Geometry check sheet. Reference: the model listing, model coordinates, mm. A direction names the side the tool comes from. Give positions to 0.01 mm unless a question says otherwise; leave off trailing zeros. Write each loop counter-clockwise with the first axis right and the second up, starting at its lowest first coordinate (ties: lowest second). Pieces come first, ordered by that corner, then holes. Notation, with made-up numbers: (8.25, 39.25) - (40.25, 39.25) arc R21 cw to (40.25, 62.25) - close; hole circle Ø10 at (-18, 39). An arc over 180 degrees is marked (long way). Write item = value, one per line. Start each with the question number.
(1) Draft check along Z on faces 1 (the cylindrical face through (23.19, -11.51, 7.57)), 2 (the flat face through (-18, 4, 41.144)), 3 (the cylindrical face through (-18.07, -11.4, 20.86)). Enter one of: pulls with the +Z half, pulls with the -Z half, needs draft (parallel to the pull), parting line crosses it, or undercut.
(2) Depth check by flat-ended pin: pin 1 Ø1.5 at (y, z) = (52.5, 6.5) entering from -X; pin 2 Ø1.1 at (x, z) = (-3.5, 0.5) entering from +Y; pin 3 Ø6 at (x, z) = (25, 34.14) entering from -Y; pin 4 Ø1 at (x, y) = (-15.5, 38.5) entering from -Z. Enter the tip coordinate at first touch or a pass-through.
(3) Thickness scan on L1, parallel to X at y = 0.5, z = 37; L2, parallel to Y at x = -28, z = 20.5; L3, parallel to Z at x = -8.5, y = 0.5. Record the ranges inside material, lowest first.
(4) Section check A-A, the plane y = 12. Enter the section's corners in (x, z).
(5) Section check D-D, the plane z = 14.5. Enter the section's corners in (x, y), plus the area to 3 significant figures.
(6) Section check B-B, the plane x = 25. Enter the section's corners in (y, z).
(7) Section check C-C, the plane y = 3. Enter the section's corners in (x, z).
(8) Access from +Z, -Z, +X, -X, +Y, -Y to the whole of each face (thin tool, end or side, straight path). Record for faces 4 (the cylindrical face through (18.1, -11.43, 20.86)), 5 (the flat face through (17.5, 25, 21)), 6 (the flat face through (33, -11, 21)), 7 (the cylindrical face through (-17.99, 26.79, 21.36)), 8 (the flat face through (-18.5, 25, 17)).
```python
from build123d import *

# Parameters (mm, degrees)
BASE_FLANGE1_DEPTH         = 1
SKETCHED_START             = -40
SKETCHED_BEND3_OUTLINE_W   = 40
SKETCHED_BEND3_OUTLINE_H   = 1
SKETCHED_BEND3_DEPTH       = 28.18876
SKETCHED_START_2           = -11.4496
SKETCHED_BEND3_2_DEPTH     = 0.4496
SKETCHED_START_3           = -12
SKETCHED_BEND3_3_DEPTH     = 2
SKETCHED_START_4           = -60
SKETCHED_BEND3_4_DEPTH     = 120
SKETCHED_BEND7_DEPTH       = 72
SKETCHED_START_5           = -10
SKETCHED_BEND7_2_OUTLINE_W = 1
SKETCHED_BEND7_2_OUTLINE_H = 40
SKETCHED_BEND7_2_DEPTH     = 55
SKETCHED_BEND7_3_DEPTH     = 20
SKETCHED_BEND7_4_DEPTH     = 2
SKETCHED_START_6           = 45
SKETCHED_BEND7_5_OUTLINE_W = 1
SKETCHED_BEND7_5_OUTLINE_H = 40
SKETCHED_BEND7_5_DEPTH     = 15
SKETCHED_START_7           = 1.14380551
SKETCHED_BEND7_6_DEPTH     = 40
SKETCHED_START_8           = -42.14380551
SKETCHED_BEND7_7_DEPTH     = 84.28761102
SKETCH9_R                  = 3
CUT_EXTRUDE1_DEPTH         = 98.989397047
F_4_CLEARANCE_HOLE1_D      = 3.2639
F_4_CLEARANCE_HOLE1_DEPTH  = 10
F_4_CLEARANCE_HOLE1_TIP    = 0.980574487
F_6_CLEARANCE_HOLE1_D      = 3.7973
F_6_CLEARANCE_HOLE2_D      = 3.7973


with BuildPart() as part:
    # Base-Flange1: sheet metal written as solids
    # Sketch1 → Base-Flange1 (new body)
    with BuildSketch(Plane.XY):
        with BuildLine():
            Line((-19, -10), (-19, -35))
            ThreePointArc((-19, -35), (-20.464466094, -38.535533906), (-24, -40))
            Line((-24, -40), (-54, -40))
            ThreePointArc((-54, -40), (-57.535533906, -38.535533906), (-59, -35))
            Line((-59, -35), (-59, 45))
            ThreePointArc((-59, 45), (-54.606601718, 55.606601718), (-44, 60))
            Line((-44, 60), (-34, 60))
            ThreePointArc((-34, 60), (-23.393398282, 55.606601718), (-19, 45))
            Line((-19, 45), (-19, 10))
            Line((-19, 10), (19, 10))
            Line((19, 10), (19, 45))
            ThreePointArc((19, 45), (23.393398282, 55.606601718), (34, 60))
            Line((34, 60), (44, 60))
            ThreePointArc((44, 60), (54.606601718, 55.606601718), (59, 45))
            Line((59, 45), (59, -35))
            ThreePointArc((59, -35), (57.535533906, -38.535533906), (54, -40))
            Line((54, -40), (24, -40))
            ThreePointArc((24, -40), (20.464466094, -38.535533906), (19, -35))
            Line((19, -35), (19, -10))
            Line((19, -10), (-19, -10))
        make_face()
    extrude(amount=-BASE_FLANGE1_DEPTH)

    # Sketched Bend3: read off the stored shape, not the designer's step
    # Sketched Bend3 outline → Sketched Bend3 (cut)
    with BuildSketch(Plane(origin=(0, 0, 0), x_dir=(1, 0, 0), z_dir=(0, 1, 0)).offset(SKETCHED_START)):
        with Locations((-39, 0.5)):
            Rectangle(SKETCHED_BEND3_OUTLINE_W, SKETCHED_BEND3_OUTLINE_H)
        with Locations((39, 0.5)):
            Rectangle(SKETCHED_BEND3_OUTLINE_W, SKETCHED_BEND3_OUTLINE_H)
    extrude(amount=SKETCHED_BEND3_DEPTH, mode=Mode.SUBTRACT)

    # Sketched Bend3 2 outline → Sketched Bend3 2 (add)
    with BuildSketch(Plane(origin=(0, 0, 0), x_dir=(1, 0, 0), z_dir=(0, 1, 0)).offset(SKETCHED_START_2)):
        with BuildLine():
            Line((-19, 1), (-19, 24.64380551))
            ThreePointArc((-19, 24.64380551), (-20.464466094, 28.179339416), (-24, 29.64380551))
            Line((-24, 29.64380551), (-54, 29.64380551))
            ThreePointArc((-54, 29.64380551), (-57.535533906, 28.179339416), (-59, 24.64380551))
            Line((-59, 24.64380551), (-59, 1))
            Line((-59, 1), (-19, 1))
        make_face()
        with BuildLine():
            Line((19, 24.64380551), (19, 1))
            Line((19, 1), (59, 1))
            Line((59, 1), (59, 24.64380551))
            ThreePointArc((59, 24.64380551), (57.535533906, 28.179339416), (54, 29.64380551))
            Line((54, 29.64380551), (24, 29.64380551))
            ThreePointArc((24, 29.64380551), (20.464466094, 28.179339416), (19, 24.64380551))
        make_face()
    extrude(amount=SKETCHED_BEND3_2_DEPTH)

    # Sketched Bend3 3 outline → Sketched Bend3 3 (add)
    with BuildSketch(Plane(origin=(0, 0, 0), x_dir=(1, 0, 0), z_dir=(0, 1, 0)).offset(SKETCHED_START_3)):
        with BuildLine():
            Line((-19, 1), (-19, 24.64380551))
            ThreePointArc((-19, 24.64380551), (-20.464466094, 28.179339416), (-24, 29.64380551))
            Line((-24, 29.64380551), (-54, 29.64380551))
            ThreePointArc((-54, 29.64380551), (-57.535533906, 28.179339416), (-59, 24.64380551))
            Line((-59, 24.64380551), (-59, 1))
            Line((-59, 1), (-19, 1))
        make_face()
        with BuildLine():
            ThreePointArc((59, 24.64380551), (57.535533906, 28.179339416), (54, 29.64380551))
            Line((54, 29.64380551), (24, 29.64380551))
            ThreePointArc((24, 29.64380551), (20.464466094, 28.179339416), (19, 24.64380551))
            Line((19, 24.64380551), (19, 1))
            Line((19, 1), (59, 1))
            Line((59, 1), (59, 24.64380551))
        make_face()
    extrude(amount=SKETCHED_BEND3_3_DEPTH)

    # Sketched Bend3 4 outline → Sketched Bend3 4 (cut)
    with BuildSketch(Plane.YZ.offset(SKETCHED_START_4)):
        with BuildLine():
            Line((-11, -2), (-11, -29.64380551))
            Line((-11, -29.64380551), (-10, -29.64380551))
            Line((-10, -29.64380551), (-10, -1))
            ThreePointArc((-10, -1), (-10.707106781, -1.292893219), (-11, -2))
        make_face()
        with BuildLine():
            Line((-12, -1), (-12, -2))
            ThreePointArc((-12, -2), (-11.414213562, -0.585786438), (-10, 0))
            Line((-10, 0), (-11.81124, 0))
            Line((-11.81124, 0), (-11.81124, -1))
            Line((-11.81124, -1), (-12, -1))
        make_face()
    extrude(amount=SKETCHED_BEND3_4_DEPTH, mode=Mode.SUBTRACT)

    # Sketched Bend7: read off the stored shape, not the designer's step
    # Sketched Bend7 outline → Sketched Bend7 (cut)
    with BuildSketch(Plane(origin=(0, 0, 0), x_dir=(1, 0, 0), z_dir=(0, 1, 0)).offset(SKETCHED_START_3)):
        with BuildLine():
            ThreePointArc((-18.232050807, 0), (-17.5, 0.732050807), (-16.5, 1))
            Line((-16.5, 1), (-19, 1))
            Line((-19, 1), (-19, 24.64380551))
            ThreePointArc((-19, 24.64380551), (-20.464466094, 28.179339416), (-24, 29.64380551))
            Line((-24, 29.64380551), (-54, 29.64380551))
            ThreePointArc((-54, 29.64380551), (-57.535533906, 28.179339416), (-59, 24.64380551))
            Line((-59, 24.64380551), (-59, 0))
            Line((-59, 0), (-18.232050807, 0))
        make_face()
        with BuildLine():
            Line((19, 1), (16.5, 1))
            ThreePointArc((16.5, 1), (17.5, 0.732050807), (18.232050807, 0))
            Line((18.232050807, 0), (59, 0))
            Line((59, 0), (59, 24.64380551))
            ThreePointArc((59, 24.64380551), (57.535533906, 28.179339416), (54, 29.64380551))
            Line((54, 29.64380551), (24, 29.64380551))
            ThreePointArc((24, 29.64380551), (20.464466094, 28.179339416), (19, 24.64380551))
            Line((19, 24.64380551), (19, 1))
        make_face()
    extrude(amount=SKETCHED_BEND7_DEPTH, mode=Mode.SUBTRACT)



with BuildPart() as body_2:
    # Sketched Bend7 2 outline → Sketched Bend7 2 (new body)
    with BuildSketch(Plane(origin=(0, 0, 0), x_dir=(1, 0, 0), z_dir=(0, 1, 0)).offset(SKETCHED_START_5)):
        with Locations((-18, -21.14380551)):
            Rectangle(SKETCHED_BEND7_2_OUTLINE_W, SKETCHED_BEND7_2_OUTLINE_H)
        with Locations((18, -21.14380551)):
            Rectangle(SKETCHED_BEND7_2_OUTLINE_W, SKETCHED_BEND7_2_OUTLINE_H)
    extrude(amount=SKETCHED_BEND7_2_DEPTH)


with BuildPart() as part_1:
    add(part.part)

    add(body_2.part)  # Sketched Bend7 3 merges body 2
    # Sketched Bend7 3 outline → Sketched Bend7 3 (add)
    with BuildSketch(Plane(origin=(0, 0, 0), x_dir=(1, 0, 0), z_dir=(0, 1, 0)).offset(SKETCHED_START_5)):
        with BuildLine():
            Line((-16.5, 0), (-18.232050807, 0))
            ThreePointArc((-18.232050807, 0), (-18.431851652, -0.48236191), (-18.5, -1))
            Line((-18.5, -1), (-18.5, -1.14380551))
            Line((-18.5, -1.14380551), (-17.5, -1.14380551))
            Line((-17.5, -1.14380551), (-17.5, -1))
            ThreePointArc((-17.5, -1), (-17.207106781, -0.292893219), (-16.5, 0))
        make_face()
        with BuildLine():
            ThreePointArc((18.5, -1), (18.431851652, -0.48236191), (18.232050807, 0))
            Line((18.232050807, 0), (16.5, 0))
            ThreePointArc((16.5, 0), (17.207106781, -0.292893219), (17.5, -1))
            Line((17.5, -1), (17.5, -1.14380551))
            Line((17.5, -1.14380551), (18.5, -1.14380551))
            Line((18.5, -1.14380551), (18.5, -1))
        make_face()
    extrude(amount=SKETCHED_BEND7_3_DEPTH)

    # Sketched Bend7 4 outline → Sketched Bend7 4 (add)
    with BuildSketch(Plane(origin=(0, 0, 0), x_dir=(1, 0, 0), z_dir=(0, 1, 0)).offset(SKETCHED_START_3)):
        with BuildLine():
            ThreePointArc((-47.14380551, -36.14380551), (-45.679339416, -39.679339416), (-42.14380551, -41.14380551))
            Line((-42.14380551, -41.14380551), (-17.5, -41.14380551))
            Line((-17.5, -41.14380551), (-17.5, -1.14380551))
            Line((-17.5, -1.14380551), (-42.14380551, -1.14380551))
            ThreePointArc((-42.14380551, -1.14380551), (-45.679339416, -2.608271604), (-47.14380551, -6.14380551))
            Line((-47.14380551, -6.14380551), (-47.14380551, -36.14380551))
        make_face()
        with BuildLine():
            ThreePointArc((42.14380551, -41.14380551), (45.679339416, -39.679339416), (47.14380551, -36.14380551))
            Line((47.14380551, -36.14380551), (47.14380551, -6.14380551))
            ThreePointArc((47.14380551, -6.14380551), (45.679339416, -2.608271604), (42.14380551, -1.14380551))
            Line((42.14380551, -1.14380551), (17.5, -1.14380551))
            Line((17.5, -1.14380551), (17.5, -41.14380551))
            Line((17.5, -41.14380551), (42.14380551, -41.14380551))
        make_face()
    extrude(amount=SKETCHED_BEND7_4_DEPTH)

    # Sketched Bend7 5 outline → Sketched Bend7 5 (add)
    with BuildSketch(Plane(origin=(0, 0, 0), x_dir=(1, 0, 0), z_dir=(0, 1, 0)).offset(SKETCHED_START_6)):
        with Locations((-18, -21.14380551)):
            Rectangle(SKETCHED_BEND7_5_OUTLINE_W, SKETCHED_BEND7_5_OUTLINE_H)
        with Locations((18, -21.14380551)):
            Rectangle(SKETCHED_BEND7_5_OUTLINE_W, SKETCHED_BEND7_5_OUTLINE_H)
    extrude(amount=SKETCHED_BEND7_5_DEPTH)

    # Sketched Bend7 6 outline → Sketched Bend7 6 (cut)
    with BuildSketch(Plane.XY.offset(SKETCHED_START_7)):
        with BuildLine():
            Line((-47.14380551, -11), (-19.5, -11))
            ThreePointArc((-19.5, -11), (-18.792893219, -10.707106781), (-18.5, -10))
            Line((-18.5, -10), (-47.14380551, -10))
            Line((-47.14380551, -10), (-47.14380551, -11))
        make_face()
        with BuildLine():
            ThreePointArc((-17.5, -10), (-18.085786438, -11.414213562), (-19.5, -12))
            Line((-19.5, -12), (-17.5, -12))
            Line((-17.5, -12), (-17.5, -10))
        make_face()
        with BuildLine():
            Line((19.5, -11), (47.14380551, -11))
            Line((47.14380551, -11), (47.14380551, -10))
            Line((47.14380551, -10), (18.5, -10))
            ThreePointArc((18.5, -10), (18.792893219, -10.707106781), (19.5, -11))
        make_face()
        with BuildLine():
            Line((17.5, -12), (19.5, -12))
            ThreePointArc((19.5, -12), (18.085786438, -11.414213562), (17.5, -10))
            Line((17.5, -10), (17.5, -12))
        make_face()
    extrude(amount=SKETCHED_BEND7_6_DEPTH, mode=Mode.SUBTRACT)

    # Sketched Bend7 7 outline → Sketched Bend7 7 (cut)
    with BuildSketch(Plane.YZ.offset(SKETCHED_START_8)):
        with BuildLine():
            ThreePointArc((45, 41.14380551), (55.606601718, 36.750407228), (60, 26.14380551))
            Line((60, 26.14380551), (60, 41.14380551))
            Line((60, 41.14380551), (45, 41.14380551))
        make_face()
        with BuildLine():
            ThreePointArc((60, 16.14380551), (55.606601718, 5.537203792), (45, 1.14380551))
            Line((45, 1.14380551), (60, 1.14380551))
            Line((60, 1.14380551), (60, 16.14380551))
        make_face()
    extrude(amount=SKETCHED_BEND7_7_DEPTH, mode=Mode.SUBTRACT)

    # Sketch9 → Cut-Extrude1 (cut, through all)
    with BuildSketch(Plane.ZY.offset(18.5)):
        with Locations(Location((21.14380551, 3, 0), (0, 0, 180))):
            Circle(SKETCH9_R)
        with Locations(Location((21.14380551, 45.4, 0), (0, 0, 180))):
            Circle(SKETCH9_R)
    extrude(amount=-CUT_EXTRUDE1_DEPTH, mode=Mode.SUBTRACT)

    # #4 Clearance Hole1
    with Locations(Plane.ZY.offset(18.5)):
        with Locations((10.93300551, 3), (31.35460551, 3), (21.14380551, 25.1742)):
            Hole(F_4_CLEARANCE_HOLE1_D / 2, depth=F_4_CLEARANCE_HOLE1_DEPTH)
            with Locations((0, 0, -(F_4_CLEARANCE_HOLE1_DEPTH + F_4_CLEARANCE_HOLE1_TIP / 2))):  # 118° drill point
                Cone(0, F_4_CLEARANCE_HOLE1_D / 2, F_4_CLEARANCE_HOLE1_TIP, mode=Mode.SUBTRACT)

    # #6 Clearance Hole1 (through all)
    with Locations(Plane.ZY.offset(18.5)):
        with Locations((11.14380551, 45.4), (31.14380551, 45.4)):
            Hole(F_6_CLEARANCE_HOLE1_D / 2)

    # #6 Clearance Hole2 (through all)
    with Locations(Plane(origin=(0, -11, 0), x_dir=(1, 0, 0), z_dir=(0, 1, 0))):
        with Locations((-40.14380551, -21.14380551), (-25, -34.14380551), (25, -34.14380551), (40.14380551, -21.14380551), (-25, -8.14380551), (25, -8.14380551)):
            Hole(F_6_CLEARANCE_HOLE2_D / 2)


solid = part_1.part
```
Model answer:
q1.face_1 = undercut
q1.face_2 = pulls with the +Z half
q1.face_3 = needs draft
q2.pin_1 = -18.5
q2.pin_2 = 10
q2.pin_3 = -12
q2.pin_4 = through
q3.L1 = -18.5 to -17.5, 17.5 to 18.5
q3.L2 = -12 to -11
q3.L3 = -1 to 0
q4.outline = (-18.5, 1.14) - (-17.5, 1.14) - (-17.5, 41.14) - (-18.5, 41.14) - close; (17.5, 1.14) - (18.5, 1.14) - (18.5, 41.14) - (17.5, 41.14) - close
q5.outline = (-47.14, -12) - (-19.5, -12) arc R2 ccw to (-17.5, -10) - (-17.5, 59.91) - (-18.5, 59.91) - (-18.5, -10) arc R1 cw to (-19.5, -11) - (-47.14, -11) - close; (17.5, -10) arc R2 ccw to (19.5, -12) - (47.14, -12) - (47.14, -11) - (19.5, -11) arc R1 cw to (18.5, -10) - (18.5, 59.91) - (17.5, 59.91) - close
q5.area = 200 mm²
q6.outline = (-12, 1.14) - (-11, 1.14) - (-11, 6.25) - (-12, 6.25) - close; (-12, 10.04) - (-11, 10.04) - (-11, 32.25) - (-12, 32.25) - close; (-12, 36.04) - (-11, 36.04) - (-11, 41.14) - (-12, 41.14) - close
q7.outline = (-18.5, 1) arc R2 ccw to (-16.5, -1) - (16.5, -1) arc R2 ccw to (18.5, 1) - (18.5, 18.14) - (17.5, 18.14) - (17.5, 1) arc R1 cw to (16.5, 0) - (-16.5, 0) arc R1 cw to (-17.5, 1) - (-17.5, 9.3) - (-18.5, 9.3) - close; (-18.5, 12.56) - (-17.5, 12.56) - (-17.5, 18.14) - (-18.5, 18.14) - close; (-18.5, 24.14) - (-17.5, 24.14) - (-17.5, 29.72) - (-18.5, 29.72) - close; (-18.5, 32.99) - (-17.5, 32.99) - (-17.5, 41.14) - (-18.5, 41.14) - close; (17.5, 24.14) - (18.5, 24.14) - (18.5, 41.14) - (17.5, 41.14) - close
q8.face_4 = +Z, -Z, -Y
q8.face_5 = +Z, +Y, -Y
q8.face_6 = +Z, -Z, +X, +Y
q8.face_7 = -X
q8.face_8 = +Z, -Z, -X, +Y
